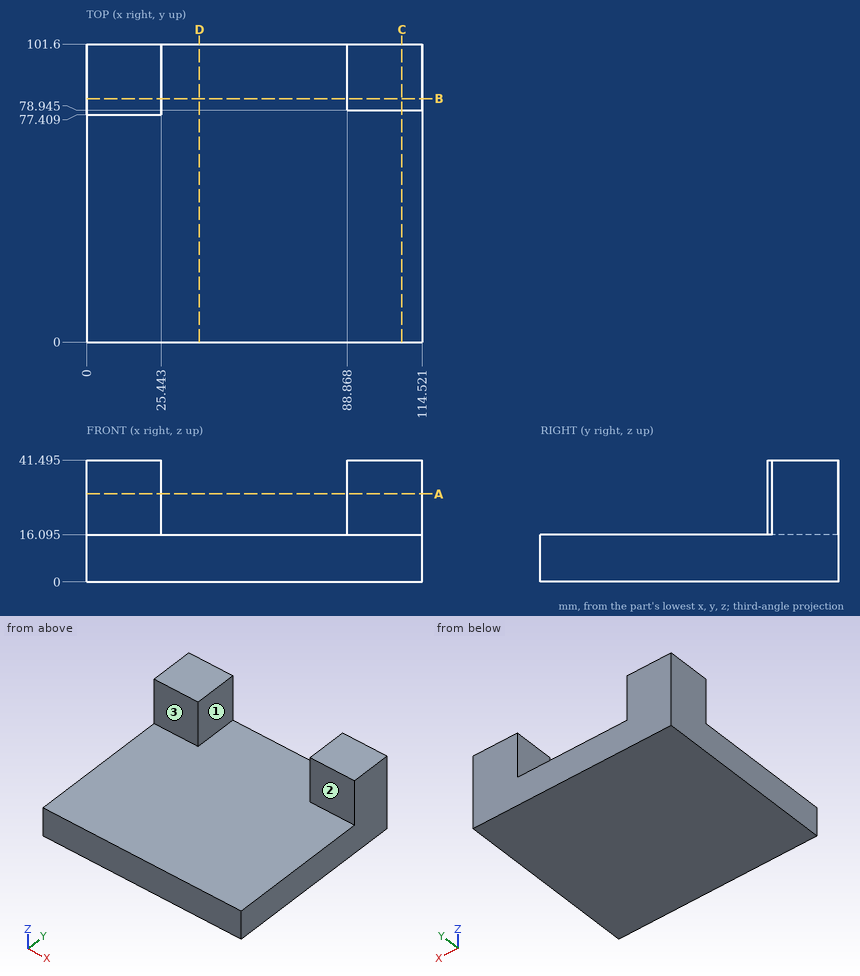
Study the drawing (mm; zero at the part's minimum x, y, z) and answer. A direction names the side the tool comes from. Give positions to 0.01 mm unless a question says otherwise; leave off trailing zeros. Loops run counter-clockwise (first coordinate to the right, second up) from the corner with the lowest first, then second, coordinate; pieces in that order, holes last. Notation, with made-up numbers: M 30,55 L 40,55 A28 ccw 40,93 Z; hole C -18.5,17.25 d6. An arc over 180 degrees is marked long. One line per item, written item: value. Start each with the question number.
1. Find section D-D (x = 38.5). Give the vertices of the cut face in (y, z) (1 decimal), and give its area (3 significant figures).
2. Find section C-C (x = 107.5). Give the vertices of the cut face in (y, z) (1 decimal), and give its area (3 significant figures).
3. Find section B-B (y = 83). Give the vertices of the cut face in (x, z) (1 decimal), and give its area (3 significant figures).
4. Find section A-A (z = 30). Give the vertices of the cut face in (x, y) (1 decimal).
5. Find the intervals of material crossed by probe 1 along X at (y, z) = (97, 37); probe 2 along Y at (x, z) = (98.5, 18) (1 decimal); probe 3 along Z at (x, y) = (21.5, 24.5) (1 decimal), in increasing order.
6. Each of these flat-tipped pins is pushed along its axis until it touches: P1, Ø12.5, axis at x = 7.5, z = 33, coming from the -Y side; P2, Ø8, axis at x = 17.5, y = 20.5, coming from the -Z side; P3, Ø12.5, axis at x = 102, z = 24, coming from the -Y side (3 decimals); P4, Ø3, axis at x = 69, z = 19, coming from the -Y side. Where does it stop, or does it pass through?
7. Which of the six approach directions +Z, -Z, +X, -X, +Y, -Y give full straight-line access (tool end or side, diameter ignored) to the marked faces 1, 2 and 3?
Reported:
1. outline: M 0,0 L 101.6,0 L 101.6,16.1 L 0,16.1 Z
1. area: 1,640 mm²
2. outline: M 0,0 L 101.6,0 L 101.6,41.5 L 78.9,41.5 L 78.9,16.1 L 0,16.1 Z
2. area: 2,210 mm²
3. outline: M 0,0 L 114.5,0 L 114.5,41.5 L 88.9,41.5 L 88.9,16.1 L 25.4,16.1 L 25.4,41.5 L 0,41.5 Z
3. area: 3,140 mm²
4. outline: M 0,77.4 L 25.4,77.4 L 25.4,101.6 L 0,101.6 Z; M 88.9,78.9 L 114.5,78.9 L 114.5,101.6 L 88.9,101.6 Z
5. probe 1: x = 0 to 25.44, 88.87 to 114.52
5. probe 2: y = 78.9 to 101.6
5. probe 3: z = 0 to 16.1
6. P1: stops at y = 77.41
6. P2: stops at z = 0
6. P3: stops at y = 78.945
6. P4: passes through
7. face 1: +Z, +Y, -Y
7. face 2: +Z, +X, -Y
7. face 3: +Z, +X, -X, -Y
